```python
from build123d import *

# Parameters (mm, degrees)
EXTRUDE_1_DEPTH              = 14
EXTRUDE_1_DEPTH_BACK         = 2
SKETCH_1_W                   = 70
SKETCH_1_H                   = 50.8
SKETCH_1_W_2                 = 64
SKETCH_1_H_2                 = 44.8
EXTRUDE_1_2_DEPTH            = 2
EXTRUDE_1_2_DEPTH_BACK       = 2
SKETCH_1_3_W                 = 17
SKETCH_1_3_H                 = 28.8
SKETCH_1_4_W                 = 17
SKETCH_1_4_H                 = 16
EXTRUDE_2_DEPTH              = 2
CUT_EXTRUDE_1_REACH          = 62.876
SKETCH_3_W                   = 20
SKETCH_3_H                   = 16
EXTRUDE_START                = -2
EXTRUDE_5_OUTLINE_W          = 10
EXTRUDE_5_OUTLINE_H          = 3
EXTRUDE_5_DEPTH              = 16
CUT_EXTRUDE_2_REACH          = 49.828
SKETCH_11_R                  = 3
CHAMFER_1_SIZE               = 1
HOLE_WIZARD_M3_1_D           = 2.5
HOLE_WIZARD_M3_1_DEPTH       = 3
HOLE_WIZARD_M3_1_CSINK_D     = 3.05
HOLE_WIZARD_M3_1_CSINK_ANGLE = 90
SKETCH_16_W                  = 50.8
SKETCH_16_H                  = 16
EXTRUDE_6_DEPTH              = 1
CUT_EXTRUDE_3_DEPTH          = 2.5


# Read off the part's stored shape, not the designer's step: M2.5 间隙孔1, 凸台-拉伸5, M3 间隙孔1
with BuildPart() as part:
    # 草图1 → Extrude 1 (new, two sides: drawn at the far end of the back side and taken through both)
    with BuildSketch(Plane(origin=(0, 0, 0), x_dir=(1, 0, 0), z_dir=(0, 1, 0)).offset(-EXTRUDE_1_DEPTH_BACK)):
        Rectangle(SKETCH_1_W, SKETCH_1_H)
        Rectangle(SKETCH_1_W_2, SKETCH_1_H_2, mode=Mode.SUBTRACT)
    extrude(amount=EXTRUDE_1_DEPTH + EXTRUDE_1_DEPTH_BACK)

    # 草图1<3> → Extrude 1 2 (add, two sides: drawn at the far end of the back side and taken through both)
    with BuildSketch(Plane(origin=(0, 0, 0), x_dir=(1, 0, 0), z_dir=(0, 1, 0)).offset(-EXTRUDE_1_2_DEPTH_BACK)):
        Polygon((32, 22.4), (15, 22.4), (15, 19.4), (29.5, 19.4), (29.5, -6.4), (32, -6.4), align=None)
        with Locations((-23.5, 8)):
            Rectangle(SKETCH_1_3_W, SKETCH_1_3_H)
    extrude(amount=EXTRUDE_1_2_DEPTH + EXTRUDE_1_2_DEPTH_BACK)

    # 草图1<4> → 凸台-拉伸2 (add)
    with BuildSketch(Plane(origin=(0, 0, 0), x_dir=(1, 0, 0), z_dir=(0, 1, 0))):
        Polygon((15, -6.4), (15, -22.4), (32, -22.4), (32, -6.4), (29.5, -6.4), align=None)
        with Locations((-23.5, -14.4)):
            Rectangle(SKETCH_1_4_W, SKETCH_1_4_H)
    extrude(amount=-EXTRUDE_2_DEPTH)

    # 草图3 → 切除-拉伸1 (cut, up to next)
    with BuildSketch(Plane(origin=(0, 0, 22.4), x_dir=(-1, 0, 0), z_dir=(0, 0, -1)), mode=Mode.PRIVATE) as cut_extrude_1_sk1:
        with Locations((-0.572922779, 6)):
            Rectangle(SKETCH_3_W, SKETCH_3_H)
    cut_extrude_1_tool1 = extrude(cut_extrude_1_sk1.sketch, amount=-CUT_EXTRUDE_1_REACH, mode=Mode.PRIVATE) & part.part
    add(cut_extrude_1_tool1.solids().sort_by_distance((0.572923, 6, 22.4))[0], mode=Mode.SUBTRACT)

    # M2.5 间隙孔1 outline → M2.5 间隙孔1 (revolve, cut)
    with BuildSketch(Plane(origin=(22, 0, 17.05), x_dir=(1, 0, 0), z_dir=(0, 0, 1))):
        Polygon((0, -2), (1.45, -2), (1.45, -0.025), (1.475, 0), (0, 0), align=None)
    revolve(axis=Axis((22, 0, 17.05), (0, 1, 0)), mode=Mode.SUBTRACT)

    # Hole Wizard M2.5 _1 2 outline → Hole Wizard M2.5 _1 2 (revolve, cut)
    with BuildSketch(Plane(origin=(-22, 0, 17.05), x_dir=(1, 0, 0), z_dir=(0, 0, 1))):
        Polygon((0, -2), (1.45, -2), (1.45, -0.025), (1.475, 0), (0, 0), align=None)
    revolve(axis=Axis((-22, 0, 17.05), (0, 1, 0)), mode=Mode.SUBTRACT)

    # 凸台-拉伸5 outline → 凸台-拉伸5 (add)
    with BuildSketch(Plane(origin=(0, 0, 0), x_dir=(1, 0, 0), z_dir=(0, 1, 0)).offset(EXTRUDE_START)):
        with Locations((0, 26.9)):
            Rectangle(EXTRUDE_5_OUTLINE_W, EXTRUDE_5_OUTLINE_H)
    extrude(amount=EXTRUDE_5_DEPTH)

    # 草图11 → 切除-拉伸2 (cut, up to next)
    with BuildSketch(Plane(origin=(0, 14, 0), x_dir=(1, 0, 0), z_dir=(0, 1, 0)), mode=Mode.PRIVATE) as cut_extrude_2_sk1:
        with Locations((0, 28.4)):
            Circle(SKETCH_11_R)
    cut_extrude_2_tool1 = extrude(cut_extrude_2_sk1.sketch, amount=-CUT_EXTRUDE_2_REACH, mode=Mode.PRIVATE) & part.part
    add(cut_extrude_2_tool1.solids().sort_by_distance((0, 14, -28.4))[0], mode=Mode.SUBTRACT)

    # 倒角1
    chamfer_1_edges = [part.edges().sort_by_distance(p)[0] for p in [
        (5, 6, -28.4),
        (-5, 6, -28.4),
        (35, 6, -25.4),
        (35, 6, 25.4),
    ]]
    chamfer(chamfer_1_edges, length=CHAMFER_1_SIZE)

    # Hole Wizard M3 _1
    with Locations(Plane(origin=(35, 0, 0), x_dir=(0, 0, -1), z_dir=(1, 0, 0))):
        with Locations((-16, 8), (16, 8)):
            CounterSinkHole(HOLE_WIZARD_M3_1_D / 2, HOLE_WIZARD_M3_1_CSINK_D / 2, depth=HOLE_WIZARD_M3_1_DEPTH, counter_sink_angle=HOLE_WIZARD_M3_1_CSINK_ANGLE)

    # 草图16 → 凸台-拉伸6 (add)
    with BuildSketch(Plane.ZY.offset(35)):
        with Locations((0, 6)):
            Rectangle(SKETCH_16_W, SKETCH_16_H)
    extrude(amount=EXTRUDE_6_DEPTH)

    # Hole Wizard M3 _1 2 outline → Hole Wizard M3 _1 2 (revolve, cut)
    with BuildSketch(Plane(origin=(0, 6, 6), x_dir=(0, 1, 0), z_dir=(0, 0, -1))):
        Polygon((1.7, -35.975), (1.7, -32), (0, -32), (0, -36), (1.725, -36), align=None)
    revolve(axis=Axis((0, 6, 6), (1, 0, 0)), mode=Mode.SUBTRACT)

    # Hole Wizard M3 _1 2 2 outline → Hole Wizard M3 _1 2 2 (revolve, cut)
    with BuildSketch(Plane(origin=(0, 6, -6), x_dir=(0, 1, 0), z_dir=(0, 0, -1))):
        Polygon((1.7, -35.975), (1.7, -32), (0, -32), (0, -36), (1.725, -36), align=None)
    revolve(axis=Axis((0, 6, -6), (1, 0, 0)), mode=Mode.SUBTRACT)

    # 草图23 → 切除-拉伸3 (cut)
    with BuildSketch(Plane(origin=(-32, 0, 0), x_dir=(0, 0, -1), z_dir=(1, 0, 0))):
        Polygon((-9.175426481, 6), (-7.58771324, 3.25), (-4.41228676, 3.25), (-2.824573519, 6), (-4.41228676, 8.75), (-7.58771324, 8.75), align=None)
        Polygon((2.824573519, 6), (4.41228676, 3.25), (7.58771324, 3.25), (9.175426481, 6), (7.58771324, 8.75), (4.41228676, 8.75), align=None)
    extrude(amount=-CUT_EXTRUDE_3_DEPTH, mode=Mode.SUBTRACT)


solid = part.part
```
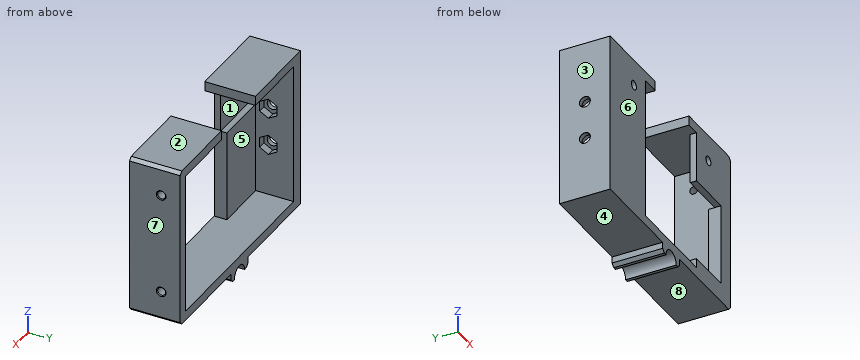
For this review, take the finished solid that the model builds, in its own axes (mm). Face numbers are marked on the shaded views. A direction names the side the tool comes from. Round coordinates to 2 decimals unless told otherwise and drop trailing zeros. Write each loop counter-clockwise with the first axis right and the second up, starting at its lowest first coordinate (ties: lowest second). Pieces come first, ordered by that corner, then holes.
1) For line 1 along X through (y, z) = (-1.35, 17.05); line 2 along Z through (x, y) = (33.05, 8); line 3 along Z through (x, y) = (22.5, 0.25), list the stretches that pass through material, from the lowest coordinate up.
Answer below:
line 1: x = -36 to -23.45, -20.55 to -15, 15 to 20.55, 23.45 to 35
line 2: z = -25.4 to -17.25, -14.75 to 14.75, 17.25 to 25.4
line 3: z = -25.4 to -19.4, 22.4 to 25.4
2) Take a section at B-B on x = 19.5. Give the boundary of the cut face in (y, z), then the cut area to 3 significant figures.
Answer below:
outline: (-2, -25.4) - (14, -25.4) - (14, -22.4) - (2, -22.4) - (2, -19.4) - (-2, -19.4) - close; (-2, 6.4) - (0, 6.4) - (0, 22.4) - (14, 22.4) - (14, 25.4) - (-2, 25.4) - close
area: 140 mm2
3) Take a section at D-D on x = -17. Give the boundary of the cut face in (y, z), then the cut area to 3 significant figures.
Answer below:
outline: (-2, -25.4) - (14, -25.4) - (14, -22.4) - (2, -22.4) - (2, 6.4) - (0, 6.4) - (0, 22.4) - (14, 22.4) - (14, 25.4) - (-2, 25.4) - close
area: 243 mm2
4) Insertion check: pin 1 Ø4.5 at (y, z) = (6, 6) entering from -X; pin 2 Ø1 at (x, y) = (20, -0.5) entering from -Z; pin 3 Ø3.5 at (x, z) = (-22, 17.05) entering from +Y; pin 4 Ø8.5 at (x, z) = (27, -13) entering from +Y. Each pin has a flat end and moves straight along its axis. Give the tip position at first contact, or say it passes through.
Answer below:
pin 1: stops at x = -36
pin 2: stops at z = -25.4
pin 3: stops at y = 0
pin 4: stops at y = 2
5) Machinability: for the marked faces 4, 5, 6, 7 and 8, which of the approach directions +Z, -Z, +X, -X, +Y, -Y give a long, thin tool a straight path to every point of the face, cutting with its end or side? Answer none if there is none.
Answer below:
face 4: -Z, -X, +Y, -Y
face 5: +Y
face 6: +Z, -Z, +X, -X, -Y
face 7: +Z, -Z, +X, +Y, -Y
face 8: -Z, +X, +Y, -Y
6) Take a section at A-A on z = -6. Give the boundary of the cut face in (x, y) (3 decimals), then the cut area to 3 significant figures.
Answer below:
outline: (-36, -2) - (-15, -2) - (-15, 2) - (-32, 2) - (-32, 3.25) - (-34.5, 3.25) - (-34.5, 4.3) - (-35.975, 4.3) - (-36, 4.275) - close; (-36, 7.725) - (-35.975, 7.7) - (-34.5, 7.7) - (-34.5, 8.75) - (-32, 8.75) - (-32, 14) - (-36, 14) - close; (29.5, -2) - (35, -2) - (35, 14) - (32, 14) - (32, 2) - (29.5, 2) - close
area: 171 mm2
7) Take a section at C-C on y = 10.5. Give the boundary of the cut face in (x, z).
Answer below:
outline: (-36, -25.4) - (-5, -25.4) - (-5, -27.4) - (-4, -28.4) - (-3, -28.4) arc R3 cw to (3, -28.4) - (4, -28.4) - (5, -27.4) - (5, -25.4) - (34, -25.4) - (35, -24.4) - (35, 24.4) - (34, 25.4) - (10.57, 25.4) - (10.57, 22.4) - (32, 22.4) - (32, -22.4) - (-32, -22.4) - (-32, 22.4) - (-9.43, 22.4) - (-9.43, 25.4) - (-36, 25.4) - close
8) Mouldability with a two-part tool opening along X and no side actions: class the marked faces 1, 2 and 3 as +X half, -X half, draft (parallel to the pull), parting line (faces both ways), or undercut.
Answer below:
face 1: undercut
face 2: draft
face 3: -X half
